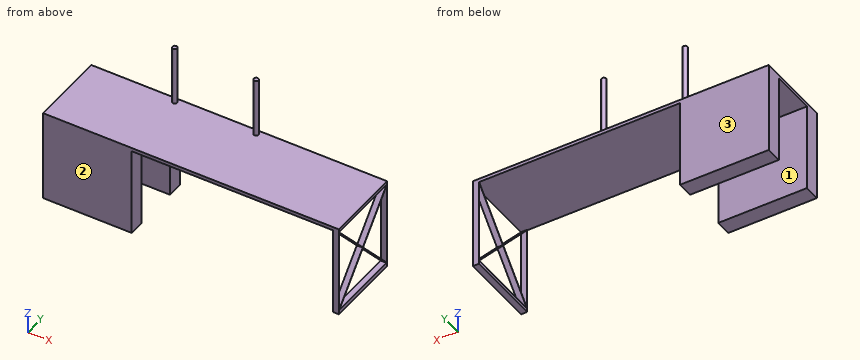
from build123d import *

# Parameters (mm, degrees)
F0_W      = 2500
F0_H      = 650
F1_DEPTH  = 30
F2_W      = 750
F2_H      = 135
F3_DEPTH  = 750
F4_W      = 50
F4_H      = 3
F5_DEPTH  = 750
F6_W      = 50
F6_H      = 30
F6_H_2    = 3
F7_DEPTH  = 644
F8_R      = 0.6
F10_R     = 20
F11_DEPTH = 500
F12_DEPTH = 50


with BuildPart() as f1:
    # F0 (on Top) → F1 (new body)
    with BuildSketch(Plane.XY):
        with Locations((15.4022108763, -104.233725491)):
            Rectangle(F0_W, F0_H)
    extrude(amount=F1_DEPTH)

    # F2 (on face) → F3 (join)
    with BuildSketch(Plane(origin=(0, 0, 0), x_dir=(1, 0, 0), z_dir=(0, 0, -1))):
        with Locations((-859.5977891237, 361.733725491)):
            Rectangle(F2_W, F2_H)
        with Locations((-859.5977891237, -153.266274509)):
            Rectangle(F2_W, F2_H)
    extrude(amount=F3_DEPTH)

    # F4 (on face) → F5 (join)
    with BuildSketch(Plane(origin=(0, 0, 0), x_dir=(1, 0, 0), z_dir=(0, 0, -1))):
        with Locations((1240.4022108763, 427.733725491)):
            Rectangle(F4_W, F4_H)
        with Locations((1240.4022108763, -219.266274509)):
            Rectangle(F4_W, F4_H)
    extrude(amount=F5_DEPTH)

    # F6 (on face) → F7 (join, through all)
    with BuildSketch(Plane(origin=(0, -426.233725491, 0), x_dir=(-1, 0, 0), z_dir=(0, 1, 0))):
        with Locations((-1240.4022108763, -735)):
            Rectangle(F6_W, F6_H)
        with Locations((-1240.4022108763, -718)):
            Rectangle(F6_W, F6_H_2)
    extrude(amount=F7_DEPTH)

    # F8
    f8_edges = [f1.edges().sort_by_distance(p)[0] for p in [
        (1215.402211, -104.233725, -716.5),
        (1215.402211, -104.233725, -719.5),
        (1265.402211, -104.233725, -719.5),
        (1265.402211, -104.233725, -716.5),
    ]]
    fillet(f8_edges, radius=F8_R)

    # F10 (on face) → F11 (join)
    with BuildSketch(Plane.XY.offset(30)):
        with Locations((-503.3661296115, 180.766274509)):
            Circle(F10_R)
        with Locations((184.1705513642, 180.766274509)):
            Circle(F10_R)
    extrude(amount=F11_DEPTH)

    # F9 (on face) → F12 (join)
    with BuildSketch(Plane.YZ.offset(1265.4022108763)):
        Polygon((-426.233725491, -2.2449458227), (-420.1270755585, -9.0447574168), (-106.2498252118, -358.55), (-426.233725491, -714.8550541773), (-426.233725491, -716.5), (-426.233725491, -717.1), (-424.2176257702, -717.1), (-104.233725491, -360.7949458227), (215.7501747882, -717.1), (217.766274509, -717.1), (217.766274509, -716.5), (217.766274509, -714.8550541773), (-102.2176257702, -358.55), (204.5102027522, -17.0057052277), (217.766274509, -2.2449458227), (217.766274509, 0), (215.7501747882, 0), (202.2781703018, -15.0012025111), (-104.233725491, -356.3050541773), (-417.8950431081, -7.0402547003), (-424.2176257702, 0), (-426.233725491, 0), align=None)
    extrude(amount=-F12_DEPTH)


solid = f1.part
Work out the finished part from the listing and answer in its coordinate system (mm). Face numbers are marked on the shaded views. Round coordinates to 2 decimals unless told otherwise and drop trailing zeros. Loops run counter-clockwise (first coordinate to the right, second up) from the corner with the lowest first, then second, coordinate; pieces in that order, holes last. Notation, with made-up numbers: M -11.5,85.25 L 18.5,85.25 A19 cw 18.5,112.25 Z; hole C -2.5,49.25 d2. An arc over 180 degrees is marked long. One line per question, with ' | ' between items. Start each with the question number.
(1) A cutting plane is placed at D-D on z = 201.5. Write down the section's boundary in (x, y).
(2) A cutting plane is placed at C-C on z = -514.5. Write down the section's boundary in (x, y), plus the area to 3 significant figures.
(3) Find the intervals of material crossed by line 1 (Y direction, x = -541.5, z = -105); line 2 (Z direction, x = 817.5, y = -174.5); line 3 (Z direction, x = -920, y = 109.5), in increasing order.
(4) A cutting plane is placed at B-B on y = -269. Write down the section's boundary in (x, z).
(5) A cutting plane is placed at A-A on x = -1048.5. Write down the section's boundary in (y, z).
(6) For a pull along Y with two mould halves and no side action, classify the marked faces 1, 2 and 3 as released by +Y, released by -Y, zero draft, split by the parting line, or undercut.
(7) Flat-ended cylindrical pins translate along their axes: pin 1 Ø2 at (x, y) = (-478.5, 50) entering from -Z; pin 2 Ø10 at (y, z) = (-289.5, -80) entering from +X. Find the tip coordinate at first contact, or state that the pin passes through.
Geometry check:
1) outline: C -503.37,180.77 d40; C 184.17,180.77 d40
2) outline: M -1234.6,-429.23 L -484.6,-429.23 L -484.6,-294.23 L -1234.6,-294.23 Z; M -1234.6,85.77 L -484.6,85.77 L -484.6,220.77 L -1234.6,220.77 Z; M 1215.4,-429.23 L 1265.4,-429.23 L 1265.4,-426.23 L 1215.4,-426.23 Z; M 1215.4,-246.3 L 1265.4,-246.3 L 1265.4,-242.27 L 1215.4,-242.27 Z; M 1215.4,33.8 L 1265.4,33.8 L 1265.4,37.84 L 1215.4,37.84 Z; M 1215.4,217.77 L 1265.4,217.77 L 1265.4,220.77 L 1215.4,220.77 Z | area: 203,000 mm²
3) line 1: y = -429.23 to -294.23, 85.77 to 220.77 | line 2: z = 0 to 30 | line 3: z = -750 to 30
4) outline: M -1234.6,0 L 1265.4,0 L 1265.4,30 L -1234.6,30 Z; M 1215.4,-750 L 1265.4,-750 L 1265.4,-720 L 1215.4,-720 Z; M 1215.4,-718.9 A0.6 ccw 1216,-719.5 L 1264.8,-719.5 A0.6 ccw 1265.4,-718.9 L 1265.4,-717.1 A0.6 ccw 1264.8,-716.5 L 1216,-716.5 A0.6 ccw 1215.4,-717.1 Z; M 1215.4,-544.26 L 1265.4,-544.26 L 1265.4,-539.77 L 1215.4,-539.77 Z; M 1215.4,-177.33 L 1265.4,-177.33 L 1265.4,-172.84 L 1215.4,-172.84 Z
5) outline: M -429.23,-750 L -294.23,-750 L -294.23,0 L 85.77,0 L 85.77,-750 L 220.77,-750 L 220.77,30 L -429.23,30 Z
6) face 1: undercut | face 2: released by -Y | face 3: released by +Y
7) pin 1: stops at z = 0 | pin 2: stops at x = -484.6
